Here's the drawing with two shaded views (mm, measured from the low corner). I have some questions. A direction names the side the tool comes from. Coordinates: 2 decimals unless noted, no trailing zeros. Write each loop counter-clockwise with the first axis right and the second up, starting at its lowest first coordinate (ties: lowest second). Pieces come first, ordered by that corner, then holes. Notation, with made-up numbers: (39, 85.5) -> (46, 85.5) arc R26 ccw to (46, 113.5) -> close; hole circle Ø6 at (67, -10). An arc over 180 degrees is marked (long way). Use a Markdown table: item, result. Add a question column.
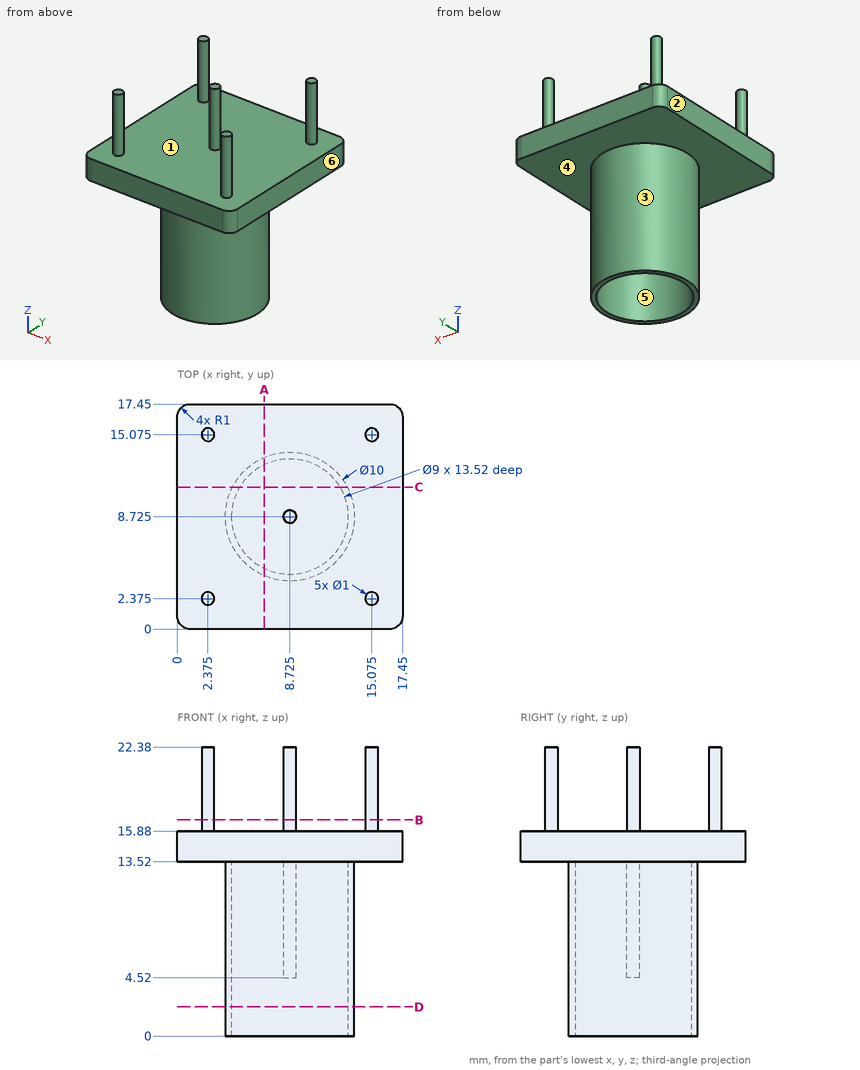
Q1. Suppose I cut it at D-D, the plane z = 2.25. Write out the boundary of the cut face in (x, y) (3 decimals), and give its area (3 significant figures).
Q2. Please list where these lines run through material, in increasing order: line 1 (Y direction, x = 8.75, z = 10.25); line 2 (Z direction, x = 2.75, y = 13); line 3 (Z direction, x = 7.25, y = 4.25).
Q3. Will these pins go through, and if not, where does the flat tip stop? pin 1 (6 mm diameter, centred on y = 3.5, z = 8, fed in from -X); pin 2 (5 mm diameter, centred on x = 13.5, z = 19.5, fed in from +Y) (3 decimals); pin 3 (3 mm diameter, centred on x = 9, z = 10.5, fed in from +Y) (3 decimals).
Q4. Thinking about a two-plate mould opening in X: for the marked faces 3, 4, 5 and 6, which applies, released by +X, released by -X, zero draft, split by the parting line, or undercut?
Q5. Suppose I cut it at C-C, the plane y = 11. Write out the boundary of the cut face in (x, z).
Q6. Suppose I cut it at A-A, the plane x = 6.75. Write out the boundary of the cut face in (y, z), and give its area (3 significant figures).
Q7. Suppose I cut it at B-B, the plane z = 16.75. Write out the boundary of the cut face in (x, y) (3 decimals), and give its area (3 significant figures).
Q8. Which directions (+Z, -Z, +X, -X, +Y, -Y) give clear straight access to the entire face, cutting with the end or side of a thin tool? Please do the marked faces 1 and 2.
Answer key:
| question | item | result |
|---|---|---|
| 1 | outline | circle Ø10 at (8.725, 8.725); hole circle Ø9 at (8.725, 8.725) |
| 1 | area | 14.9 mm^2 |
| 2 | line 1 | y = 3.73 to 4.23, 8.23 to 9.22, 13.22 to 13.72 |
| 2 | line 2 | z = 13.52 to 15.88 |
| 2 | line 3 | z = 0 to 15.88 |
| 3 | pin 1 | stops at x = 4.25 |
| 3 | pin 2 | stops at y = 15.575 |
| 3 | pin 3 | stops at y = 13.725 |
| 4 | face 3 | split by the parting line |
| 4 | face 4 | zero draft |
| 4 | face 5 | undercut |
| 4 | face 6 | released by +X |
| 5 | outline | (0, 13.52) -> (4.27, 13.52) -> (4.27, 0) -> (4.84, 0) -> (4.84, 13.52) -> (12.61, 13.52) -> (12.61, 0) -> (13.18, 0) -> (13.18, 13.52) -> (17.45, 13.52) -> (17.45, 15.88) -> (0, 15.88) -> close |
| 6 | outline | (0, 13.52) -> (4.13, 13.52) -> (4.13, 0) -> (4.68, 0) -> (4.68, 13.52) -> (12.77, 13.52) -> (12.77, 0) -> (13.32, 0) -> (13.32, 13.52) -> (17.45, 13.52) -> (17.45, 15.88) -> (0, 15.88) -> close |
| 6 | area | 56.1 mm^2 |
| 7 | outline | circle Ø1 at (2.375, 2.375); circle Ø1 at (2.375, 15.075); circle Ø1 at (8.725, 8.725); circle Ø1 at (15.075, 2.375); circle Ø1 at (15.075, 15.075) |
| 7 | area | 3.93 mm^2 |
| 8 | face 1 | +Z |
| 8 | face 2 | +Z, -Z, -X, +Y, -Y |
